Design review of the part shown in the three views and the two pictorial views. Dimensions are in mm from the part's minimum x, y and z. Give positions to 0.01 mm unless a question says otherwise; leave off trailing zeros. Write each loop counter-clockwise with the first axis right and the second up, starting at its lowest first coordinate (ties: lowest second). Pieces come first, ordered by that corner, then holes. Notation, with made-up numbers: M 80,3 L 123,3 A25 ccw 123,38 Z; hole C -0.5,47 d11. An arc over 180 degrees is marked long. Write item = value, one per line.
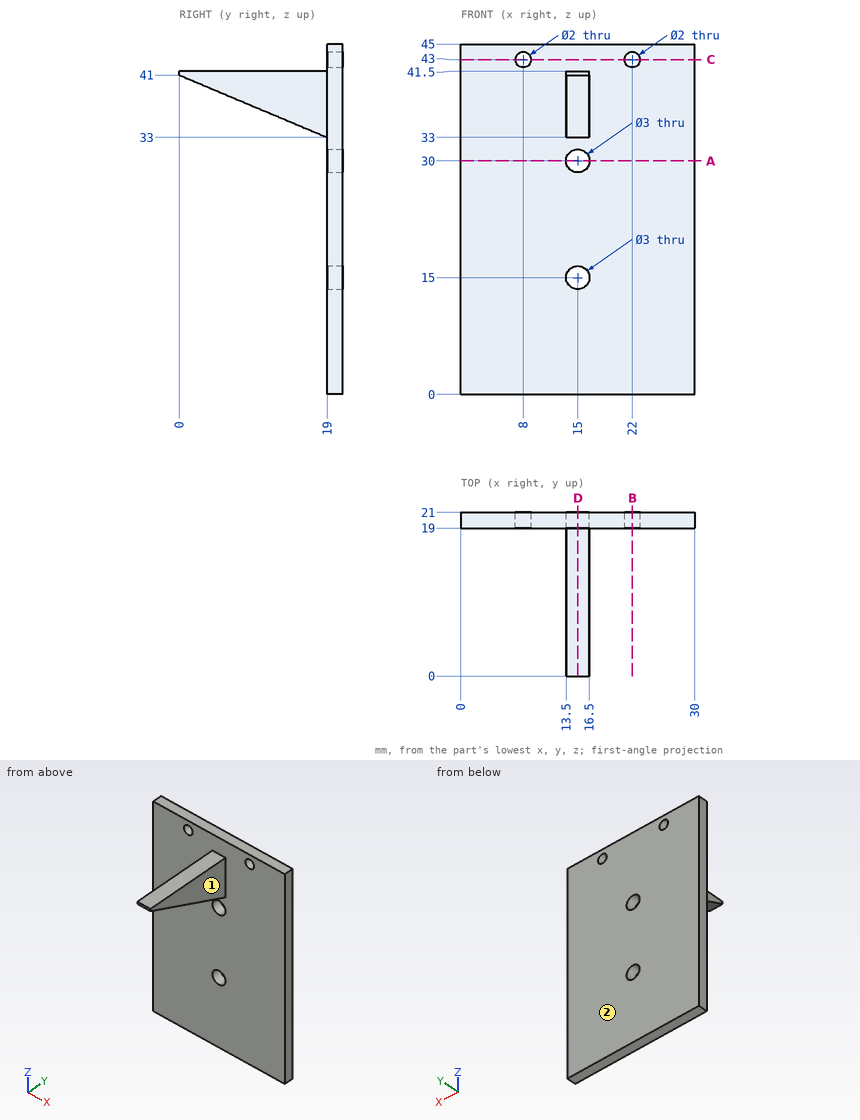
1. We need section A-A, the plane z = 30. Write out the cut boundary in (x, y), then the cut area to 3 significant figures.
Responses:
outline = M 0,19 L 13.5,19 L 13.5,21 L 0,21 Z; M 16.5,19 L 30,19 L 30,21 L 16.5,21 Z
area = 54.0 mm2
2. Insertion check: P1, Ø12, axis at x = 15.5, y = 2.5, coming from the +Z side; P2, Ø1.8, axis at x = 15, z = 15, coming from the -Y side; P3, Ø4, axis at y = 6, z = 38.5, coming from the -X side; P4, Ø9.5, axis at y = 12.5, z = 37, coming from the +X side. Each pin has a flat end and moves straight along its axis. Give the tip position at first contact, or say it passes through.
Responses:
P1 = 41.5
P2 = through
P3 = 13.5
P4 = 16.5
3. We need section D-D, the plane x = 15. Count the separate pieces of the cut face and the enclosed holes in it, then the cut area to 4 significant figures.
Responses:
separate_pieces = 3
enclosed_holes = 0
area = 163.5 mm2
4. We need section B-B, the plane x = 22. Write out the cut boundary in (y, z), then the cut area to 3 significant figures.
Responses:
outline = M 19,0 L 21,0 L 21,42 L 19,42 Z; M 19,44 L 21,44 L 21,45 L 19,45 Z
area = 86.0 mm2
5. For line 1 along Z through (x, y) = (15, 19.9); line 2 along Z through (x, y) = (8, 19.6); line 3 along Y through (x, z) = (23.5, 15.5), list the stretches that pass through material, from the lowest coordinate up. Write a range as from..to.
Responses:
line_1 = 0..13.5, 16.5..28.5, 31.5..45
line_2 = 0..42, 44..45
line_3 = 19..21
6. The part is to be moulded in two halves that separate along Y. For the marked faces 1 and 2, say which applies: +Y half, -Y half, draft (parallel to the pull), parting line (faces both ways), or undercut.
Responses:
face_1 = draft
face_2 = +Y half
7. We need section C-C, the plane z = 43. Write out the cut boundary in (x, y).
Responses:
outline = M 0,19 L 7,19 L 7,21 L 0,21 Z; M 9,19 L 21,19 L 21,21 L 9,21 Z; M 23,19 L 30,19 L 30,21 L 23,21 Z
